```python
from build123d import *

# Parameters (mm, degrees)
SKETCH1_W           = 50
SKETCH1_H           = 50
SKETCH1_R           = 11.15
SKETCH1_R_2         = 2.15
SKETCH1_R_3         = 1.65
BOSS_EXTRUDE1_DEPTH = 4
BOSS_EXTRUDE2_START = 42
SKETCH2_W           = 12
SKETCH2_H           = 12
SKETCH2_R           = 2.15
BOSS_EXTRUDE2_DEPTH = 42
CHAMFER1_SIZE       = 2.5
CUT_EXTRUDE1_START  = -8
SKETCH3_R           = 4.5
CUT_EXTRUDE1_DEPTH  = 51.017238817
SKETCH5_W           = 56
SKETCH5_H           = 56
CUT_EXTRUDE2_DEPTH  = 55.899908925
BOSS_EXTRUDE3_DEPTH = 4
CIRPATTERN1_COUNT   = 4


with BuildPart() as part:
    # Sketch1 → Boss-Extrude1 (new body)
    with BuildSketch(Plane.XY):
        Rectangle(SKETCH1_W, SKETCH1_H)
        Circle(SKETCH1_R, mode=Mode.SUBTRACT)
        with Locations((-17, 17)):
            Circle(SKETCH1_R_2, mode=Mode.SUBTRACT)
        with Locations((17, 17)):
            Circle(SKETCH1_R_2, mode=Mode.SUBTRACT)
        with Locations((17, -17)):
            Circle(SKETCH1_R_2, mode=Mode.SUBTRACT)
        with Locations((-17, -17)):
            Circle(SKETCH1_R_2, mode=Mode.SUBTRACT)
        with Locations((-21.920310217, 0)):
            Circle(SKETCH1_R_3, mode=Mode.SUBTRACT)
        with Locations((0, 21.920310217)):
            Circle(SKETCH1_R_3, mode=Mode.SUBTRACT)
        with Locations((21.920310217, 0)):
            Circle(SKETCH1_R_3, mode=Mode.SUBTRACT)
        with Locations((0, -21.920310217)):
            Circle(SKETCH1_R_3, mode=Mode.SUBTRACT)
    extrude(amount=-BOSS_EXTRUDE1_DEPTH)

    # Sketch2 → Boss-Extrude2 (add)
    # profile 1 of 4: a face of its own
    with BuildSketch(Plane.XY.offset(BOSS_EXTRUDE2_START)):
        with Locations((-17, 17)):
            Rectangle(SKETCH2_W, SKETCH2_H)
        with Locations((-17, 17)):
            Circle(SKETCH2_R, mode=Mode.SUBTRACT)
    # profile 2 of 4: a face of its own
    with BuildSketch(Plane.XY.offset(BOSS_EXTRUDE2_START)):
        with Locations((17, 17)):
            Rectangle(SKETCH2_W, SKETCH2_H)
        with Locations((17, 17)):
            Circle(SKETCH2_R, mode=Mode.SUBTRACT)
    # profile 3 of 4: a face of its own
    with BuildSketch(Plane.XY.offset(BOSS_EXTRUDE2_START)):
        with Locations((17, -17)):
            Rectangle(SKETCH2_W, SKETCH2_H)
        with Locations((17, -17)):
            Circle(SKETCH2_R, mode=Mode.SUBTRACT)
    # profile 4 of 4: a face of its own
    with BuildSketch(Plane.XY.offset(BOSS_EXTRUDE2_START)):
        with Locations((-17, -17)):
            Rectangle(SKETCH2_W, SKETCH2_H)
        with Locations((-17, -17)):
            Circle(SKETCH2_R, mode=Mode.SUBTRACT)
    extrude(amount=-BOSS_EXTRUDE2_DEPTH)

    # Chamfer1
    chamfer1_edges = [part.edges().sort_by_distance(p)[0] for p in [
        (-23, 23, 21),
        (-23, 11, 21),
        (-11, 11, 21),
        (-11, 23, 21),
        (23, 11, 21),
        (23, 23, 21),
        (11, 23, 21),
        (11, 11, 21),
        (23, -23, 21),
        (23, -11, 21),
        (11, -11, 21),
        (11, -23, 21),
        (-23, -11, 21),
        (-23, -23, 21),
        (-11, -23, 21),
        (-11, -11, 21),
    ]]
    chamfer(chamfer1_edges, length=CHAMFER1_SIZE)

    # Sketch3 → Cut-Extrude1 (cut, through all)
    with BuildSketch(Plane.XY.offset(42).offset(CUT_EXTRUDE1_START)):
        with Locations((-17, 17)):
            Circle(SKETCH3_R)
        with Locations((17, 17)):
            Circle(SKETCH3_R)
        with Locations((17, -17)):
            Circle(SKETCH3_R)
        with Locations((-17, -17)):
            Circle(SKETCH3_R)
    extrude(amount=-CUT_EXTRUDE1_DEPTH, mode=Mode.SUBTRACT)

    # Sketch5 → Cut-Extrude2 (cut, through all)
    with BuildSketch(Plane.XY):
        Rectangle(SKETCH5_W, SKETCH5_H)
        Polygon((-23, 20.5), (-20.5, 23), (-13.5, 23), (-6, 25), (6, 25), (13.5, 23), (20.5, 23), (23, 20.5), (23, 13.5), (25, 6), (25, -6), (23, -13.5), (23, -20.5), (20.5, -23), (13.5, -23), (6, -25), (-6, -25), (-13.5, -23), (-20.5, -23), (-23, -20.5), (-23, -13.5), (-25, -6), (-25, 6), (-23, 13.5), align=None, mode=Mode.SUBTRACT)
    extrude(amount=-CUT_EXTRUDE2_DEPTH, mode=Mode.SUBTRACT)

    # Sketch6 → Boss-Extrude3 (add)
    with BuildSketch(Plane.XY):
        Polygon((-6, 25), (-1.5, 26.2), (1.5, 26.2), (6, 25), align=None)
    boss_extrude3 = extrude(amount=-BOSS_EXTRUDE3_DEPTH)

    # CirPattern1: Boss-Extrude3 ×4 about axis
    cirpattern1_axis = Axis((0, 0, 0), (0, 0, 1))
    for i in range(1, CIRPATTERN1_COUNT):
        add(boss_extrude3.rotate(cirpattern1_axis, i * 360 / CIRPATTERN1_COUNT))


solid = part.part
```
Part model, mm, in its own coordinate system. A direction names the side the tool comes from. Coordinates: 2 decimals unless noted, no trailing zeros. Loops run counter-clockwise (first coordinate to the right, second up) from the corner with the lowest first, then second, coordinate; pieces in that order, holes last. Notation, with made-up numbers: (80.5, 37) - (139.5, 37) arc R27 cw to (139.5, 62) - close; hole circle Ø9 at (46, 65.25). An arc over 180 degrees is marked (long way). Write item = value, one per line. Start each with the question number.
Item 1: Cut at A-A, the plane y = 0. Give the cut face in (x, z).
Item 2: Cut at C-C, the plane y = 17. Give the cut face in (x, z), and give its area (3 significant figures).
Item 3: Cut at D-D, the plane z = 25.5. State how many separate pieces and enclosed holes the cut face has, and give its area (3 significant figures).
Item 4: Flat gauge pins, fed straight in: pin 1 Ø2 at (x, z) = (-18, 16) entering from -Y; pin 2 Ø7.5 at (y, z) = (-17.5, 10.5) entering from +X; pin 3 Ø4.5 at (x, y) = (-21.92, 0) entering from +Z; pin 4 Ø8 at (x, z) = (-3.5, 17) entering from -Y. Where does each tip first touch, or does it go through?
Item 5: Wall check: L1, parallel to Y at x = -17, z = 16; L2, parallel to Y at x = -17, z = 37; L3, parallel to X at y = -14, z = 25.5. Give the ranges that are in metal, low to high. Write a range as from..to.
Item 6: 3-axis set-ups, long thin cutter, end or side, ignore diameter. For faces 4 (the cylindrical face through (13.68, -13.96, 15.27)), 5 (the flat face through (17, 11, 21)), 6 (the flat face through (-11, -17, 21)), 7 (the flat face through (-12.3, 12.2, 21.3)): which of +Z, -Z, +X, -X, +Y, -Y reach the whole face in a straight line?
Item 7: Mould opens along X. For faces 1 (the flat face through (12.3, 12.2, 21.3)), 2 (the flat face through (23, 17, 19)), 3 (the flat face through (-14, 17, 42)) say: released by +X, released by -X, zero draft, split by the parting line, or undercut.
The answers:
q1.outline = (-26.2, -4) - (-23.57, -4) - (-23.57, 0) - (-26.2, 0) - close; (-20.27, -4) - (-11.15, -4) - (-11.15, 0) - (-20.27, 0) - close; (11.15, -4) - (20.27, -4) - (20.27, 0) - (11.15, 0) - close; (23.57, -4) - (26.2, -4) - (26.2, 0) - (23.57, 0) - close
q2.outline = (-23, -4) - (-21.5, -4) - (-21.5, 34) - (-19.15, 34) - (-19.15, 42) - (-23, 42) - close; (-14.85, 34) - (-12.5, 34) - (-12.5, -4) - (12.5, -4) - (12.5, 34) - (14.85, 34) - (14.85, 42) - (11, 42) - (11, 0) - (-11, 0) - (-11, 42) - (-14.85, 42) - close; (19.15, 34) - (21.5, 34) - (21.5, -4) - (23, -4) - (23, 42) - (19.15, 42) - close
q2.area = 439 mm2
q3.separate_pieces = 4
q3.enclosed_holes = 4
q3.area = 272 mm2
q4.pin_1 = -23
q4.pin_2 = 23
q4.pin_3 = 0
q4.pin_4 = through
q5.L1 = -23..-21.5, -12.5..-11, 11..12.5, 21.5..23
q5.L2 = -23..-19.15, -14.85..-11, 11..14.85, 19.15..23
q5.L3 = -23..-20.35, -13.65..-11, 11..13.65, 20.35..23
q6.face_4 = -Z
q6.face_5 = +Z, +X, -X
q6.face_6 = +Z, +Y, -Y
q6.face_7 = +Z
q7.face_1 = undercut
q7.face_2 = released by +X
q7.face_3 = zero draft
